```python
from build123d import *

# Parameters (mm, degrees)
F0_W     = 19.05
F0_H     = 12.7
F2_R     = 12.7
F3_DEPTH = 6.35
F4_W     = 14.3478936436
F4_H     = 5.08
F5_DEPTH = 6.35


# Not quite as in the source:
# - a feature of the source that left no trace in its solid (it failed there, or was rolled back) is left out


with BuildPart() as f1:
    # F0 (on Front) → F1 (revolve)
    with BuildSketch(Plane.XZ):
        with Locations((9.525, 50.8)):
            Rectangle(F0_W, F0_H)
        with BuildLine():
            Line((0, 44.45), (0, 0))
            Line((0, 0), (19.05, 0))
            Line((19.05, 0), (19.05, 12.7))
            add(Edge.make_bspline(
                [(19.05, 12.7), (16.3044854864, 14.4605922783), (11.5816284357, 18.1369797007), (8.0678489786, 26.6218092545), (8.7605074506, 39.8132017689), (17.6573194939, 42.2227860015), (19.05, 44.45)],
                knots=[0, 0, 0, 0, 0.2386598147, 0.4768090303, 0.7479827182, 1, 1, 1, 1], degree=3))
            Line((19.05, 44.45), (0, 44.45))
        make_face()
    revolve(axis=Axis((0, 0, 28.575), (0, 0, 1)))

    # F2 (on face) → F3 (cut)
    with BuildSketch(Plane.XY.offset(57.15)):
        Circle(F2_R)
    extrude(amount=-F3_DEPTH, mode=Mode.SUBTRACT)

    # F4 (on face) → F5 (cut)
    with BuildSketch(Plane.XY.offset(57.15)):
        with Locations((19.05, 0)):
            Rectangle(F4_W, F4_H)
        Polygon((11.1008845043, 4.9257238661), (22.7085742955, 13.3592041513), (19.7226252138, 17.4690104828), (8.1149354226, 9.0355301976), align=None)
        Polygon((6.0855174874, 10.5099886346), (10.5192604568, 24.1556463795), (5.687893354, 25.7254527109), (1.2541503846, 12.079794966), align=None)
        Polygon((-1.2543481381, 12.079794966), (-5.6880911074, 25.7254527109), (-10.5194582102, 24.1556463795), (-6.0857152409, 10.5099886346), align=None)
        Polygon((-8.1151331761, 9.0355301976), (-19.7228229673, 17.4690104828), (-22.7087720489, 13.3592041513), (-11.1010822577, 4.9257238661), align=None)
        with Locations((-19.0501977534, 0)):
            Rectangle(F4_W, F4_H)
        Polygon((-11.1010822577, -4.9257238661), (-22.7087720489, -13.3592041513), (-19.7228229673, -17.4690104828), (-8.1151331761, -9.0355301976), align=None)
        Polygon((-6.0857152409, -10.5099886346), (-10.5194582102, -24.1556463795), (-5.6880911074, -25.7254527109), (-1.2543481381, -12.079794966), align=None)
        Polygon((1.2541503846, -12.079794966), (5.687893354, -25.7254527109), (10.5192604568, -24.1556463795), (6.0855174874, -10.5099886346), align=None)
        Polygon((8.1149354226, -9.0355301976), (19.7226252138, -17.4690104828), (22.7085742955, -13.3592041513), (11.1008845043, -4.9257238661), align=None)
    extrude(amount=-F5_DEPTH, mode=Mode.SUBTRACT)


solid = f1.part
```
CAD build for the part. Positions are in the model's coordinates, mm. A direction names the side the tool comes from. Coordinates: 2 decimals unless noted, no trailing zeros. Write each loop counter-clockwise with the first axis right and the second up, starting at its lowest first coordinate (ties: lowest second). Pieces come first, ordered by that corner, then holes. Notation, with made-up numbers: (-21.5, 47.25) -> (3.5, 47.25) arc R15 ccw to (3.5, 69.25) -> close; hole circle Ø4 at (12, 72.5). An arc over 180 degrees is marked (long way). Use CSV: the item, a comma, the result in double quotes. Start each with the question number.
Item 1: Tool access for faces 1 (the flat face through (11.214, 11.287, 54.019)), 2 (the flat face through (-11.214, -11.287, 54.019)), 3 (the flat face through (16, 2.54, 54)), 4 (the cylindrical face through (0, 12.7, 54)): list every direction of +Z, -Z, +X, -X, +Y, -Y with a clear straight run to the whole face (end or side of a thin tool).
Item 2: Band-saw the part on A-A, the plane z = 9.5. Write the cut outline in (x, y).
Item 3: Drop flat-ended pins along their axis: P1, Ø7, axis at x = 16.5, z = 54, coming from the -Y side; P2, Ø3, axis at x = 9.5, z = 35.5, coming from the -Y side; P3, Ø5, axis at y = 2, z = 32.5, coming from the -X side. Give the stop position or say it passes through.
Item 4: Wall check: probe 1 along Y at (x, z) = (-12.5, 53.5); probe 2 along Z at (x, y) = (5.5, 4); probe 3 along X at (y, z) = (9.5, 51.5). Give the ranges that are in metal, low to high.
Item 5: Two-plate mould, pull along Y, no slides. Class faces 5 (the flat face through (14.2, -7.177, 54.019)), 6 (the flat face through (0, 17, 57.15)), 7 (the flat face through (7.241, 14.067, 54.019)): +Y half, -Y half, draft (parallel to the pull), parting line (faces both ways), or undercut.
Response values:
1,face 1,"+Z, +X"
1,face 2,"+Z, -X"
1,face 3,"+Z, +X, -X"
1,face 4,"+Z"
2,outline,"circle Ø38.1 at (0, 0)"
3,P1,"stops at y = -13.92"
3,P2,"stops at y = -5.21"
3,P3,"stops at x = -9.13"
4,probe 1,"y = -14.38 to -12.22, -5.94 to -2.54, 2.54 to 5.94, 12.22 to 14.38"
4,probe 2,"z = 0 to 50.8"
4,probe 3,"x = -8.75 to -8.43, 8.43 to 8.75"
5,face 5,"undercut"
5,face 6,"draft"
5,face 7,"+Y half"
